```python
from build123d import *

# Parameters (mm, degrees)
PLENUM_BACKPLATE_START  = -57
SKETCH_1_R              = 80
SKETCH_1_R_2            = 23
PLENUM_BACKPLATE_DEPTH  = 2
PLENUM_OUTER_WALL_START = -57
SKETCH_2_R              = 80
SKETCH_2_R_2            = 78
PLENUM_OUTER_WALL_DEPTH = 8
PLENUM_INNER_WALL_START = -57
SKETCH_3_R              = 25
SKETCH_3_R_2            = 23
PLENUM_INNER_WALL_DEPTH = 8
SKETCH_4_R              = 23
THROUGH_HOLES_DEPTH     = 100


with BuildPart() as part:
    # Эскиз1 → Plenum_backplate (new body)
    with BuildSketch(Plane.XY.offset(PLENUM_BACKPLATE_START)):
        Circle(SKETCH_1_R)
        Circle(SKETCH_1_R_2, mode=Mode.SUBTRACT)
    extrude(amount=PLENUM_BACKPLATE_DEPTH)

    # Эскиз2 → Plenum_outer_wall (add)
    with BuildSketch(Plane.XY.offset(PLENUM_OUTER_WALL_START)):
        Circle(SKETCH_2_R)
        Circle(SKETCH_2_R_2, mode=Mode.SUBTRACT)
    extrude(amount=PLENUM_OUTER_WALL_DEPTH)

    # Эскиз3 → Plenum_inner_wall (add)
    with BuildSketch(Plane.XY.offset(PLENUM_INNER_WALL_START)):
        Circle(SKETCH_3_R)
        Circle(SKETCH_3_R_2, mode=Mode.SUBTRACT)
    extrude(amount=PLENUM_INNER_WALL_DEPTH)

    # Эскиз4 → Through_holes (cut, symmetric)
    with BuildSketch(Plane.XY):
        with Locations((-48, 0)):
            Circle(SKETCH_4_R)
        with Locations((48, 0)):
            Circle(SKETCH_4_R)
    extrude(amount=THROUGH_HOLES_DEPTH, both=True, mode=Mode.SUBTRACT)


solid = part.part
```
Here's how the part is built. I have some questions about the finished solid (model axes, mm). A direction names the side the tool comes from. Round coordinates to 2 decimals unless told otherwise and drop trailing zeros. Write each loop counter-clockwise with the first axis right and the second up, starting at its lowest first coordinate (ties: lowest second). Pieces come first, ordered by that corner, then holes.
Q1. Will these pins go through, and if not, where does the flat tip stop? P1, Ø1.5, axis at y = -28, z = -54, coming from the +X side; P2, Ø8, axis at x = 21.5, y = 57, coming from the +Z side; P3, Ø1, axis at x = 26.5, z = -53, coming from the -Y side.
Q2. Please list where these lines run through material, in increasing order: probe 1 along Y at (x, z) = (0, -52.8); probe 2 along Y at (x, z) = (-9, -53); probe 3 along X at (y, z) = (-14, -53.75).
Q3. If we section it at D-D on y = 28.5: Write out the boundary of the cut face in (x, z).
Q4. If we mould it in two halves opening along Y, with no side actions, what happens to faces 1 (the flat face through (22.1, -7.3, -49)), 2 (the cylindrical face through (-2.994, 22.804, -53.056)), 3 (the cylindrical face through (-17.34, -78.1, -53.06))? For each: +Y half, -Y half, draft (parallel to the pull), parting line (faces both ways), or undercut.
Q5. If we section it at A-A on z = -53: Write out the boundary of the cut face in (x, y), plus the area to 3 significant figures.
Q6. Which directions (+Z, -Z, +X, -X, +Y, -Y) give clear straight access to the entire face, cutting with the end or side of a thin tool? Please do faces 4 (the cylindrical face through (23.846, 7.509, -52.042)), 5 (the flat face through (77, -17, -49)).
Q7. If we section it at B-B on x = 18: Write out the boundary of the cut face in (y, z), plus the area to 3 significant figures.
Q8. If we section it at C-C on y = -18.5: Write out the boundary of the cut face in (x, z).
Answer below:
1. P1: stops at x = 75.22
1. P2: stops at z = -55
1. P3: stops at y = -75.66
2. probe 1: y = -80 to -78, -25 to -23, 23 to 25, 78 to 80
2. probe 2: y = -79.49 to -77.48, -23.32 to -21.17, 21.17 to 23.32, 77.48 to 79.49
2. probe 3: x = -78.77 to -76.73, -20.71 to -18.25, 18.25 to 20.71, 76.73 to 78.77
3. outline: (-74.75, -57) - (74.75, -57) - (74.75, -49) - (72.61, -49) - (72.61, -55) - (-72.61, -55) - (-72.61, -49) - (-74.75, -49) - close
4. face 1: draft
4. face 2: undercut
4. face 3: parting line
5. outline: circle Ø160 at (0, 0); circle Ø50 at (0, 0); hole circle Ø156 at (0, 0); hole circle Ø46 at (0, 0)
5. area: 1,290 mm2
6. face 4: +Z
6. face 5: +Z, +X, -X, +Y, -Y
7. outline: (-77.95, -57) - (-14.32, -57) - (-14.32, -49) - (-17.35, -49) - (-17.35, -55) - (-75.89, -55) - (-75.89, -49) - (-77.95, -49) - close; (14.32, -57) - (77.95, -57) - (77.95, -49) - (75.89, -49) - (75.89, -55) - (17.35, -55) - (17.35, -49) - (14.32, -49) - close
7. area: 316 mm2
8. outline: (-77.83, -57) - (-61.67, -57) - (-61.67, -55) - (-75.77, -55) - (-75.77, -49) - (-77.83, -49) - close; (-34.33, -57) - (-13.67, -57) - (-13.67, -49) - (-16.82, -49) - (-16.82, -55) - (-34.33, -55) - close; (13.67, -57) - (34.33, -57) - (34.33, -55) - (16.82, -55) - (16.82, -49) - (13.67, -49) - close; (61.67, -57) - (77.83, -57) - (77.83, -49) - (75.77, -49) - (75.77, -55) - (61.67, -55) - close
